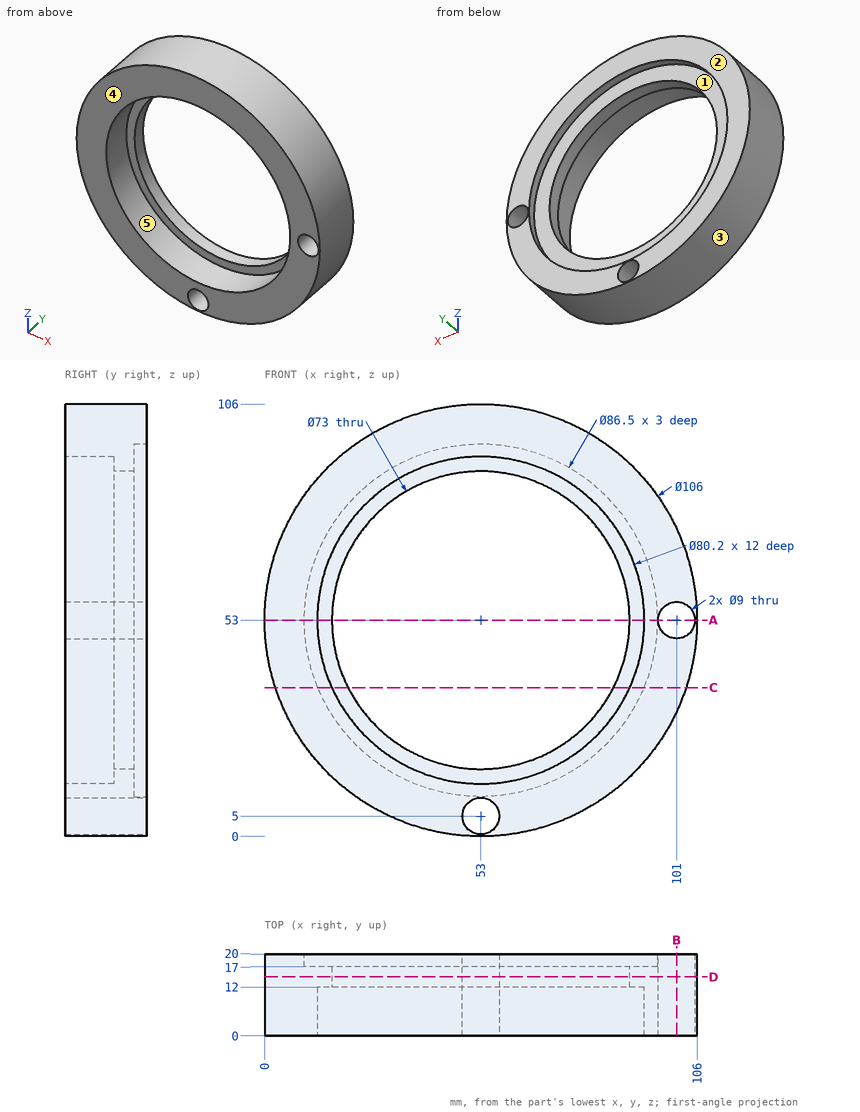
Part print with two shaded views. Sizes in mm from the minimum x, y, z corner. A direction names the side the tool comes from. Round coordinates to 2 decimals unless told otherwise and drop trailing zeros. Order: outer loops, then holes, each group sorted by start corner. A loop starts at its lowest first (then second) coordinate and runs counter-clockwise, first axis right, second up. Notation, with made-up numbers: M 74,-33.5 L 82,-33.5 A7 cw 82,-24.5 Z; hole C -18,12.25 d1. An arc over 180 degrees is marked long. Answer in a Markdown table with one row per item. Add a question column.
Q1. Cut at A-A on z = 53. Give the cut face in (x, y), and give its area (3 significant figures).
Q2. Cut at C-C on z = 36.5. Give the cut face in (x, y), and give its area (3 significant figures).
Q3. Cut at B-B on x = 101. Give the cut face in (y, z), and give its area (3 significant figures).
Q4. 3-axis set-ups, long thin cutter, end or side, ignore diameter. For the marked faces 1 and 2: which of +Z, -Z, +X, -X, +Y, -Y reach the whole face in a straight line?
Q5. Pin check, flat tips, straight feed: pin 1 (12 mm diameter, centred on y = 17, z = 76.5, fed in from +X); pin 2 (8 mm diameter, centred on x = 48, z = 86.5, fed in from -Y); pin 3 (5.5 mm diameter, centred on x = 53, z = 5, fed in from -Y); pin 4 (12 mm diameter, centred on x = 35.5, y = 17, fed in from -Z). Stop position of each tip, or through.
Q6. Wall check: L1, parallel to Z at x = 53, y = 9; L2, parallel to X at y = 18.15, z = 53; L3, parallel to Z at x = 53, y = 18.05. Give the ranges that are in metal, low to high. Write a range as from..to.
Q7. Cut at D-D on y = 14.5. Give the cut face in (x, z), and give its area (3 significant figures).
Q8. Mould opens along X. For the marked faces 3, 4 and 5 say: +X half, -X half, draft (parallel to the pull), parting line (faces both ways), or undercut.
Established:
| question | item | result |
|---|---|---|
| 1 | outline | M 0,0 L 12.9,0 L 12.9,12 L 16.5,12 L 16.5,17 L 9.75,17 L 9.75,20 L 0,20 Z; M 89.5,12 L 93.1,12 L 93.1,0 L 96.5,0 L 96.5,20 L 96.25,20 L 96.25,17 L 89.5,17 Z; M 105.5,0 L 106,0 L 106,20 L 105.5,20 Z |
| 1 | area | 353 mm2 |
| 2 | outline | M 2.63,0 L 16.45,0 L 16.45,12 L 20.44,12 L 20.44,17 L 13.02,17 L 13.02,20 L 2.63,20 Z; M 85.56,12 L 89.55,12 L 89.55,0 L 103.37,0 L 103.37,20 L 92.98,20 L 92.98,17 L 85.56,17 Z |
| 2 | area | 572 mm2 |
| 3 | outline | M 0,30.53 L 20,30.53 L 20,48.5 L 0,48.5 Z; M 0,57.5 L 20,57.5 L 20,75.47 L 0,75.47 Z |
| 3 | area | 719 mm2 |
| 4 | face 1 | +Y |
| 4 | face 2 | +Z, -Z, +X, -X, +Y |
| 5 | pin 1 | stops at x = 103.03 |
| 5 | pin 2 | stops at y = 12 |
| 5 | pin 3 | passes through |
| 5 | pin 4 | stops at z = 1.26 |
| 6 | L1 | z = 0..0.5, 9.5..12.9, 93.1..106 |
| 6 | L2 | x = 0..9.75, 96.25..96.5, 105.5..106 |
| 6 | L3 | z = 0..0.5, 9.5..9.75, 96.25..106 |
| 7 | outline | C 53,53 d106; hole C 53,53 d73; hole C 53,5 d9; hole C 101,53 d9 |
| 7 | area | 4,510 mm2 |
| 8 | face 3 | parting line |
| 8 | face 4 | draft |
| 8 | face 5 | undercut |
